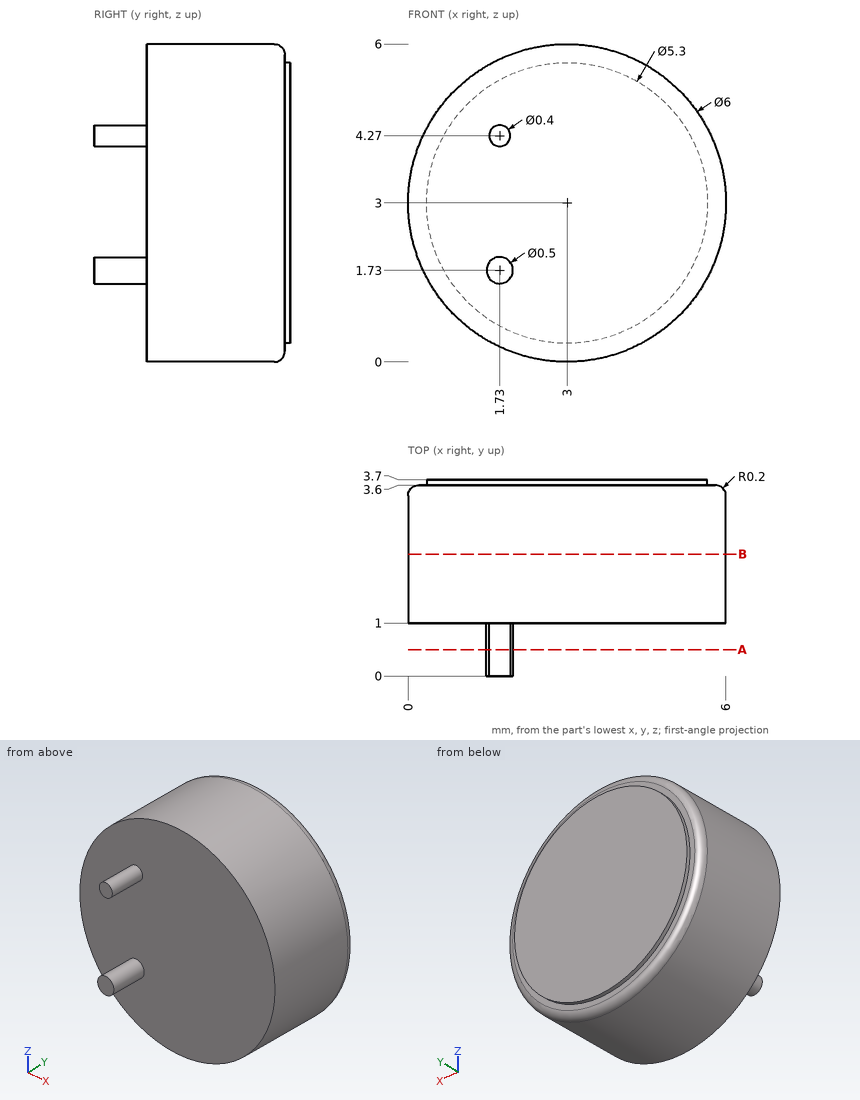
Can you work these out from the drawing? Everything is in mm from the part's minimum corner. Round coordinates to 2 decimals unless told otherwise and drop trailing zeros. Write each loop counter-clockwise with the first axis right and the second up, starting at its lowest first coordinate (ties: lowest second). Pieces come first, ordered by that corner, then holes. Notation, with made-up numbers: M 56.25,-33.5 L 114.25,-33.5 A21 cw 114.25,-4.5 Z; hole C -3.75,66.25 d5. An arc over 180 degrees is marked long. Use a Markdown table: item, result.
Item 1: I want a section at A-A (y = 0.5). List the corners of the cut face in (x, z) for me.
Found:
| item | result |
|---|---|
| outline | C 1.73,1.73 d0.5; C 1.73,4.27 d0.4 |
Item 2: I want a section at B-B (y = 2.3). List the corners of the cut face in (x, z) for me.
Found:
| item | result |
|---|---|
| outline | C 3,3 d6 |
Item 3: If I drill on line 1 along Y through (x, z) = (5.5, 3); line 2 along Y through (x, z) = (1.5, 5.25); line 3 along Z through (x, y) = (1, 1.4), over which ranges is the centre line in solid material (lowest first)? Write a range as [from, to].
Found:
| item | result |
|---|---|
| line 1 | y = [1, 3.7] |
| line 2 | y = [1, 3.6] |
| line 3 | z = [0.76, 5.24] |
Item 4: For pin 1 Ø1.5 at (x, y) = (4, 1.5) entering from +Z, with a flat end and sliding along its axis, tell me the tip position at first contact or that it passes through.
Found:
| item | result |
|---|---|
| pin 1 | stops at z = 5.99 |
